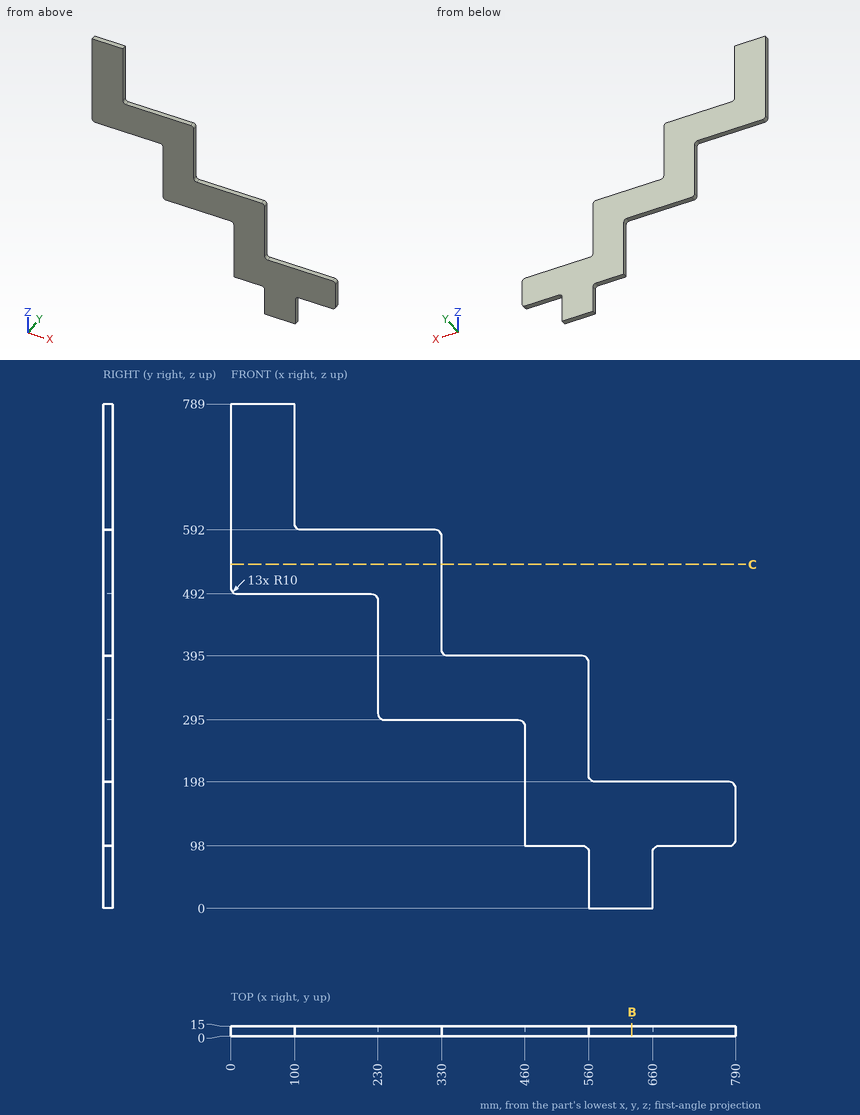
Job drawing, mm, ordinate dimensions from the low corner. One solid piece. Round coordinates to 2 decimals unless told otherwise and drop trailing zeros. Write each loop counter-clockwise with the first axis right and the second up, starting at its lowest first coordinate (ties: lowest second). Pieces come first, ordered by that corner, then holes. Notation, with made-up numbers: (-39, -35) -> (6, -35) arc R15 cw to (6, -17) -> close; hole circle Ø1 at (74.25, -32.5). An arc over 180 degrees is marked (long way). Answer as a JSON object with one key per item and string values.
(1) Pin check, flat tips, straight feed: P1, Ø7.5, axis at x = 158.5, y = 11, coming from the -Z side; P2, Ø7.5, axis at x = 495, y = 7.5, coming from the +Z side; P3, Ø5, axis at y = 4, z = 616, coming from the +X side. Stop position of each tip, or through.
Reported:
{"P1": "stops at z = 492", "P2": "stops at z = 395", "P3": "stops at x = 100"}
(2) Band-saw the part on B-B, the plane x = 627.5. List the corners of the cut face in (y, z).
Reported:
{"outline": "(0, 0) -> (15, 0) -> (15, 198) -> (0, 198) -> close"}
(3) Band-saw the part on C-C, the plane z = 538. List the corners of the cut face in (x, y), then the cut area to 3 significant figures.
Reported:
{"outline": "(0, 0) -> (330, 0) -> (330, 15) -> (0, 15) -> close", "area": "4,950 mm^2"}
(4) Probe probe 1 along X at (y, z) = (12.75, 383); probe 2 along Z at (x, y) = (300.5, 10.5); probe 3 along X at (y, z) = (0.5, 534). List the from-to ranges inside material, lowest first. Write a range as [from, to].
Reported:
{"probe 1": "x = [230, 560]", "probe 2": "z = [295, 592]", "probe 3": "x = [0, 330]"}
